from build123d import *

# Parameters (mm, degrees)
SKETCH1_W           = 40
SKETCH1_H           = 62
BOSS_EXTRUDE1_DEPTH = 25
CUT_EXTRUDE1_DEPTH  = 25
SKETCH3_R           = 4
CUT_EXTRUDE2_DEPTH  = 30


with BuildPart() as part:
    # Sketch1 → Boss-Extrude1 (new body)
    with BuildSketch(Plane.XY):
        Rectangle(SKETCH1_W, SKETCH1_H)
    extrude(amount=BOSS_EXTRUDE1_DEPTH)

    # Sketch2 → Cut-Extrude1 (cut)
    with BuildSketch(Plane.XY.offset(25)):
        Polygon((0, -31), (-20, -11), (-20, -38.533016332), (20, -38.533016332), (20, -11), align=None)
    extrude(amount=-CUT_EXTRUDE1_DEPTH, mode=Mode.SUBTRACT)

    # Sketch3 → Cut-Extrude2 (cut)
    with BuildSketch(Plane(origin=(0, 31, 0), x_dir=(1, 0, 0), z_dir=(0, 1, 0))):
        with Locations((0, -12.5)):
            Circle(SKETCH3_R)
    extrude(amount=-CUT_EXTRUDE2_DEPTH, mode=Mode.SUBTRACT)


solid = part.part
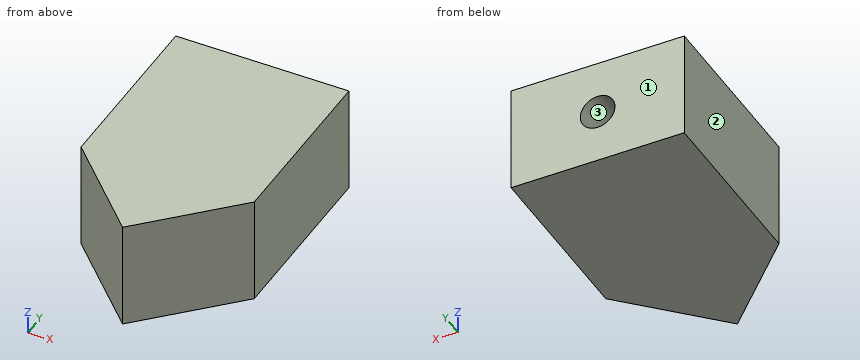
Verification items for the finished model (mm, model axes). Face numbers are marked on the shaded views. Round coordinates to 2 decimals unless told otherwise and drop trailing zeros. Loops run counter-clockwise (first coordinate to the right, second up) from the corner with the lowest first, then second, coordinate; pieces in that order, holes last. Notation, with made-up numbers: (-35.5, 55) - (17.5, 55) arc R23 ccw to (17.5, 70) - close; hole circle Ø4 at (-3, 2.5). An arc over 180 degrees is marked (long way). Answer in a Markdown table with one row per item. Add a question column.
Q1. Gauge pin test, flat ends, axial feed: pin 1 (3 mm diameter, centred on x = 10, y = -7, fed in from -Z); pin 2 (12 mm diameter, centred on y = -19.5, z = 18, fed in from -X); pin 3 (4 mm diameter, centred on y = -21.5, z = 9.5, fed in from -X); pin 4 (3 mm diameter, centred on x = -9, z = 13.5, fed in from -Y). Record the tip position at first contact, or that the pin passes through.
Q2. Section check C-C on y = -22.5. Enter the section's corners in (x, z).
Q3. Section check A-A on z = 12.5. Enter the section's corners in (x, y), plus the area to 3 significant figures.
Q4. Section check D-D on x = 2. Enter the section's corners in (y, z).
Q5. Release check for a two-part mould opening along X. For the marked faces 1, 2 and 3 record: pulls with the +X half, pulls with the -X half, needs draft (parallel to the pull), parting line crosses it, or undercut.
Q6. Material ranges on line 1 (X direction, y = 14, z = 12.5); line 2 (Z direction, x = 0, y = 8.5); line 3 (Y direction, x = -14, z = 19.5), recorded low to high.
Q7. Section check B-B on y = 3. Enter the section's corners in (x, z), plus the area to 3 significant figures.
Found:
| question | item | result |
|---|---|---|
| 1 | pin 1 | stops at z = 0 |
| 1 | pin 2 | stops at x = -17.5 |
| 1 | pin 3 | stops at x = -11.5 |
| 1 | pin 4 | stops at y = -23.5 |
| 2 | outline | (-8.5, 0) - (8.5, 0) - (8.5, 25) - (-8.5, 25) - close |
| 3 | outline | (-20, -11) - (0, -31) - (20, -11) - (20, 31) - (4, 31) - (4, 1) - (-4, 1) - (-4, 31) - (-20, 31) - close |
| 3 | area | 1,840 mm² |
| 4 | outline | (-29, 0) - (31, 0) - (31, 9.04) - (1, 9.04) - (1, 15.96) - (31, 15.96) - (31, 25) - (-29, 25) - close |
| 5 | face 1 | needs draft |
| 5 | face 2 | pulls with the -X half |
| 5 | face 3 | undercut |
| 6 | line 1 | x = -20 to -4, 4 to 20 |
| 6 | line 2 | z = 0 to 8.5, 16.5 to 25 |
| 6 | line 3 | y = -17 to 31 |
| 7 | outline | (-20, 0) - (20, 0) - (20, 25) - (-20, 25) - close; hole circle Ø8 at (0, 12.5) |
| 7 | area | 950 mm² |
